For this review, take the finished solid that the model builds, in its own axes (mm). Give positions to 0.01 mm unless a question says otherwise; leave off trailing zeros. Answer in a Markdown table with one row per item.
```python
from build123d import *

# Parameters (mm, degrees)
SKETCH1_R      = 3.399999999
EXTRUDE1_DEPTH = 300


with BuildPart() as part:
    # Sketch1 → Extrude1 (new body)
    with BuildSketch(Plane.XY):
        with BuildLine():
            Line((-2.059593866, -18.104416256), (8.279174121, -18.104416256))
            ThreePointArc((8.279174121, -18.104416256), (11.181313383, -16.857158108), (12.273594224, -13.893210106))
            ThreePointArc((12.273594224, -13.893210106), (9.65925826, 2.588190449), (3.682639337, 18.16867))
            ThreePointArc((3.682639337, 18.16867), (1.25472238, 20.189383847), (-1.882233023, 19.818471458))
            Line((-1.882233023, 19.818471458), (-10.835868733, 14.649087471))
            ThreePointArc((-10.835868733, 14.649087471), (-11.517306455, 13.688428826), (-11.352775107, 12.522173349))
            Line((-11.352775107, 12.522173349), (-10.895632574, 11.730379256))
            ThreePointArc((-10.895632574, 11.730379256), (-9.971755302, 11.005610738), (-8.804122697, 11.130000122))
            Line((-8.804122697, 11.130000122), (-8.137309536, 11.51498488))
            ThreePointArc((-8.137309536, 11.51498488), (-7.962051999, 11.739304298), (-7.991807639, 12.022410299))
            Line((-7.991807639, 12.022410299), (-8.005205154, 12.04760736))
            ThreePointArc((-8.005205154, 12.04760736), (-8.034960793, 12.33071336), (-7.859703256, 12.555032779))
            Line((-7.859703256, 12.555032779), (-6.204847981, 13.510463917))
            ThreePointArc((-6.204847981, 13.510463917), (-5.241268241, 13.637321596), (-4.470212547, 13.045669753))
            Line((-4.470212547, 13.045669753), (-3.250166277, 10.932487626))
            ThreePointArc((-3.250166277, 10.932487626), (-3.138682315, 10.604066463), (-3.161365902, 10.257981807))
            Line((-3.161365902, 10.257981807), (-4.364267951, 5.768690249))
            ThreePointArc((-4.364267951, 5.768690249), (-5.183850297, 4.106741659), (-6.577045843, 2.884941957))
            Line((-6.577045843, 2.884941957), (-12.432727244, -0.495837277))
            ThreePointArc((-12.432727244, -0.495837277), (-14.187434599, -1.091480161), (-16.036515473, -0.970284996))
            Line((-16.036515473, -0.970284996), (-20.52580703, 0.232617053))
            ThreePointArc((-20.52580703, 0.232617053), (-20.836866927, 0.386014818), (-21.065546016, 0.646773342))
            Line((-21.065546016, 0.646773342), (-22.285592286, 2.75995547))
            ThreePointArc((-22.285592286, 2.75995547), (-22.412449965, 3.72353521), (-21.820798122, 4.494590904))
            Line((-21.820798122, 4.494590904), (-20.165942847, 5.450022043))
            ThreePointArc((-20.165942847, 5.450022043), (-19.884047763, 5.489639813), (-19.653748594, 5.322317672))
            Line((-19.653748594, 5.322317672), (-19.638626056, 5.298116553))
            ThreePointArc((-19.638626056, 5.298116553), (-19.408326887, 5.130794413), (-19.126431804, 5.170412183))
            Line((-19.126431804, 5.170412183), (-18.514604376, 5.523650914))
            ThreePointArc((-18.514604376, 5.523650914), (-17.78095609, 6.479759973), (-17.938259613, 7.674598851))
            Line((-17.938259613, 7.674598851), (-18.39540247, 8.466393505))
            ThreePointArc((-18.39540247, 8.466393505), (-19.35151153, 9.200041791), (-20.546350407, 9.042738268))
            Line((-20.546350407, 9.042738268), (-29.662040307, 3.779792251))
            ThreePointArc((-29.662040307, 3.779792251), (-31.47445664, 1.526261453), (-31.294110083, -1.360038798))
            ThreePointArc((-31.294110083, -1.360038798), (-28.977774789, -7.764571351), (-27.781513715, -14.469226888))
            ThreePointArc((-27.781513715, -14.469226888), (-26.49454829, -17.059009504), (-23.798184307, -18.104416256))
            Line((-23.798184307, -18.104416256), (-13.272292278, -18.104416256))
            ThreePointArc((-13.272292278, -18.104416256), (-12.158879696, -17.643225664), (-11.697689104, -16.529813082))
            Line((-11.697689104, -16.529813082), (-11.697689104, -15.615527367))
            ThreePointArc((-11.697689104, -15.615527367), (-12.158879696, -14.502114785), (-13.272292278, -14.040924193))
            Line((-13.272292278, -14.040924193), (-13.978769739, -14.040924193))
            ThreePointArc((-13.978769739, -14.040924193), (-14.242706928, -14.147561739), (-14.358490788, -14.407616548))
            Line((-14.358490788, -14.407616548), (-14.35948673, -14.4361366))
            ThreePointArc((-14.35948673, -14.4361366), (-14.475270591, -14.696191409), (-14.739207779, -14.802828955))
            Line((-14.739207779, -14.802828955), (-16.650070056, -14.802828955))
            ThreePointArc((-16.650070056, -14.802828955), (-17.547983429, -14.430901058), (-17.919911326, -13.532987685))
            Line((-17.919911326, -13.532987685), (-17.919911326, -11.092895145))
            ThreePointArc((-17.919911326, -11.092895145), (-17.852248688, -10.752732094), (-17.659561798, -10.464355784))
            Line((-17.659561798, -10.464355784), (-14.373172288, -7.177966273))
            ThreePointArc((-14.373172288, -7.177966273), (-12.83241886, -6.148467746), (-11.014976273, -5.786955939))
            Line((-11.014976273, -5.786955939), (-4.253417808, -5.786955939))
            ThreePointArc((-4.253417808, -5.786955939), (-2.435975221, -6.148467746), (-0.895221793, -7.177966273))
            Line((-0.895221793, -7.177966273), (2.391167718, -10.464355784))
            ThreePointArc((2.391167718, -10.464355784), (2.583854608, -10.752732094), (2.651517245, -11.092895145))
            Line((2.651517245, -11.092895145), (2.651517245, -13.532987685))
            ThreePointArc((2.651517245, -13.532987685), (2.279589349, -14.430901058), (1.381675976, -14.802828955))
            Line((1.381675976, -14.802828955), (-0.529186301, -14.802828955))
            ThreePointArc((-0.529186301, -14.802828955), (-0.79312349, -14.696191409), (-0.90890735, -14.4361366))
            Line((-0.90890735, -14.4361366), (-0.909903292, -14.407616548))
            ThreePointArc((-0.909903292, -14.407616548), (-1.025687153, -14.147561739), (-1.289624342, -14.040924193))
            Line((-1.289624342, -14.040924193), (-2.059593866, -14.040924193))
            ThreePointArc((-2.059593866, -14.040924193), (-3.132988051, -14.517016132), (-3.570704977, -15.606622714))
            Line((-3.570704977, -15.606622714), (-3.570704977, -16.520908428))
            ThreePointArc((-3.570704977, -16.520908428), (-3.130065344, -17.61318056), (-2.059593866, -18.104416256))
        make_face()
        with Locations((3.2e-08, -5.5e-08)):
            Circle(SKETCH1_R, mode=Mode.SUBTRACT)
        with BuildLine():
            Line((-17.471996997, -2.585491548), (-16.423939067, -6.496897212))
            ThreePointArc((-16.423939067, -6.496897212), (-16.409679865, -6.826087675), (-16.53608811, -7.130374779))
            ThreePointArc((-16.53608811, -7.130374779), (-17.543650961, -8.076355418), (-18.844475383, -8.543172397))
            ThreePointArc((-18.844475383, -8.543172397), (-19.312155652, -8.797217087), (-19.498513244, -9.29574932))
            Line((-19.498513244, -9.29574932), (-19.498513244, -15.662799546))
            ThreePointArc((-19.498513244, -15.662799546), (-19.718246677, -16.197319926), (-20.250387025, -16.4227561))
            Line((-20.250387025, -16.4227561), (-23.778549311, -16.460482754))
            ThreePointArc((-23.778549311, -16.460482754), (-25.37859993, -15.854783364), (-26.143910087, -14.324641508))
            ThreePointArc((-26.143910087, -14.324641508), (-27.389825963, -7.33908176), (-29.803611037, -0.666451621))
            ThreePointArc((-29.803611037, -0.666451621), (-29.905903927, 1.041345175), (-28.823069139, 2.365921544))
            Line((-28.823069139, 2.365921544), (-25.748727644, 4.097330446))
            ThreePointArc((-25.748727644, 4.097330446), (-25.175162497, 4.168167167), (-24.717607571, 3.815125655))
            Line((-24.717607571, 3.815125655), (-21.534082474, -1.698901561))
            ThreePointArc((-21.534082474, -1.698901561), (-21.123425948, -2.037464343), (-20.591380608, -2.023633363))
            ThreePointArc((-20.591380608, -2.023633363), (-19.231425073, -1.777496514), (-17.885859686, -2.092958393))
            ThreePointArc((-17.885859686, -2.092958393), (-17.624243388, -2.293274639), (-17.471996997, -2.585491548))
        make_face(mode=Mode.SUBTRACT)
        with BuildLine():
            Line((7.190897434, 0.242092847), (7.722900865, 0.38464274))
            ThreePointArc((7.722900865, 0.38464274), (8.309684208, 0.302794353), (8.659411124, -0.175436695))
            ThreePointArc((8.659411124, -0.175436695), (9.953652351, -7.035721769), (10.632131313, -13.983976078))
            ThreePointArc((10.632131313, -13.983976078), (9.981645181, -15.73436744), (8.260122506, -16.457804934))
            Line((8.260122506, -16.457804934), (5.002311314, -16.422756139))
            ThreePointArc((5.002311314, -16.422756139), (4.47017203, -16.197320416), (4.250439036, -15.662801104))
            Line((4.250439036, -15.662801104), (4.250439036, -9.395167615))
            ThreePointArc((4.250439036, -9.395167615), (4.192587481, -9.104328206), (4.02784019, -8.857766461))
            Line((4.02784019, -8.857766461), (2.472174548, -7.302100819))
            ThreePointArc((2.472174548, -7.302100819), (2.262321312, -6.626096356), (2.700649697, -6.070318845))
            ThreePointArc((2.700649697, -6.070318845), (5.448190239, -3.80256528), (6.629279814, -0.441507013))
            ThreePointArc((6.629279814, -0.441507013), (6.800365527, -0.009563085), (7.190897434, 0.242092847))
        make_face(mode=Mode.SUBTRACT)
        with BuildLine():
            Line((-1.510084411, 7.559891942), (-0.940671266, 9.684970729))
            ThreePointArc((-0.940671266, 9.684970729), (-0.921276799, 9.980873109), (-1.016595587, 10.261673203))
            Line((-1.016595587, 10.261673203), (-4.150412332, 15.689603027))
            ThreePointArc((-4.150412332, 15.689603027), (-4.227383934, 16.262352796), (-3.879292116, 16.723654228))
            Line((-3.879292116, 16.723654228), (-1.075426501, 18.382938276))
            ThreePointArc((-1.075426501, 18.382938276), (0.77717457, 18.617184399), (2.215707781, 17.426544162))
            ThreePointArc((2.215707781, 17.426544162), (5.102254892, 11.069940004), (7.411551633, 4.48163831))
            ThreePointArc((7.411551633, 4.48163831), (7.347794829, 3.892614543), (6.8805497, 3.528340035))
            Line((6.8805497, 3.528340035), (6.348546228, 3.385790132))
            ThreePointArc((6.348546228, 3.385790132), (5.884507712, 3.408464604), (5.520371172, 3.696996155))
            ThreePointArc((5.520371172, 3.696996155), (2.816988485, 6.017213134), (-0.69632814, 6.607375035))
            ThreePointArc((-0.69632814, 6.607375035), (-1.353820412, 6.869528286), (-1.510084411, 7.559891942))
        make_face(mode=Mode.SUBTRACT)
        with BuildLine():
            Line((-6.519522932, -4.269206071), (-13.09653484, -4.269206071))
            ThreePointArc((-13.09653484, -4.269206071), (-13.830638522, -3.705908495), (-13.476534864, -2.851026646))
            Line((-13.476534864, -2.851026646), (-7.780675483, 0.437479301))
            ThreePointArc((-7.780675483, 0.437479301), (-7.030528407, 0.443070393), (-6.641013202, -0.198045665))
            ThreePointArc((-6.641013202, -0.198045665), (-6.417577923, -1.719584898), (-5.850308929, -3.148994163))
            ThreePointArc((-5.850308929, -3.148994163), (-5.867080961, -3.89897456), (-6.519522932, -4.269206071))
        make_face(mode=Mode.SUBTRACT)
    extrude(amount=-EXTRUDE1_DEPTH)


solid = part.part
```
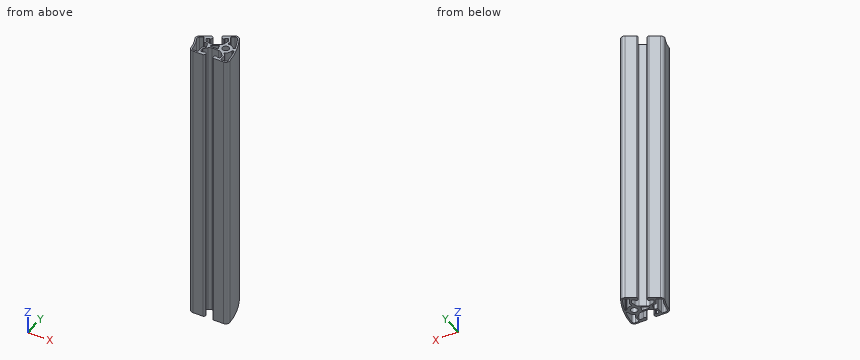
1. Clearance check with flat-ended pins moving along their axes: pin 1 (3 mm diameter, centred on x = -9.5, y = 3, fed in from +Z); pin 2 (0.6 mm diameter, centred on x = -15, z = -151.5, fed in from +Y); pin 3 (8 mm diameter, centred on x = 0, y = 0, fed in from -Z); pin 4 (0.5 mm diameter, centred on y = -16, z = -171.5, fed in from +X) (3 decimals). State where each tip first meets the part, or that it passes through.
Values:
| item | result |
|---|---|
| pin 1 | passes through |
| pin 2 | stops at y = -1.11 |
| pin 3 | stops at z = -300 |
| pin 4 | stops at x = 11.925 |
2. We need section A-A, the plane z = -209.5. Count the separate pieces of the cut face and the enclosed holes in it, and give its area (3 significant figures).
Values:
| item | result |
|---|---|
| separate pieces | 1 |
| enclosed holes | 5 |
| area | 472 mm^2 |
3. Wall thickness on line 1 (Y direction, x = 0, z = -88); line 2 (Y direction, x = -19, z = -52); line 3 (Y direction, x = -22, z = -115.5): over which ranges is each line inside the solid? List them lowest first. Write a range as [from, to].
Values:
| item | result |
|---|---|
| line 1 | y = [-18.1, -14.8], [-8.07, -3.4], [3.4, 6.64], [18.71, 20.35] |
| line 2 | y = [-18.1, -8.58], [-1.79, -0.18], [5.24, 9.06] |
| line 3 | y = [-18.1, -16.44], [-0.89, 2.27], [4.37, 8.2] |
